Job drawing, mm, ordinate dimensions from the low corner. One solid piece. A direction names the side the tool comes from. Give positions to 0.01 mm unless a question says otherwise; leave off trailing zeros. Write each loop counter-clockwise with the first axis right and the second up, starting at its lowest first coordinate (ties: lowest second). Pieces come first, ordered by that corner, then holes. Notation, with made-up numbers: (-2, -7.5) -> (31, -7.5) arc R13 cw to (31, 17.5) -> close; hole circle Ø10 at (5, 22). An arc over 180 degrees is marked (long way). Put each result on its own line as item: value. Start each with the question number.
Item 1: Flat gauge pins, fed straight in: pin 1 Ø4 at (y, z) = (9, 18.5) entering from -X; pin 2 Ø1.9 at (x, z) = (34, 19) entering from -Y; pin 3 Ø1 at (x, z) = (14.5, 12.5) entering from -Y. Where does each tip first touch, or does it go through?
Item 2: Slice it at A-A, the plane x = 3.81. List the corners of the cut face in (y, z) (1 decimal).
Item 3: Two-plate mould, pull along X, no slides. Class the marked faces 3, 4 and 5: pulls with the +X half, pulls with the -X half, needs draft (parallel to the pull), parting line crosses it, or undercut.
Item 4: Slice it at B-B, the plane z = 15.5. List the corners of the cut face in (x, y).
Item 5: Slice it at C-C, the plane y = 5. Give the number of separate pieces and of enclosed holes in the cut face.
Item 6: Tool access for the marked faces 1 and 2: list every direction of +Z, -Z, +X, -X, +Y, -Y with a clear straight run to the whole face (end or side of a thin tool).
Item 7: Drill centre lines: line 1 along Z through (x, y) = (16, 2.75) (1 decimal); line 2 along Z through (x, y) = (3.81, 14) (1 decimal); line 3 along X through (y, z) = (6.5, 22.75). Where is each one in solid material? Low to high.
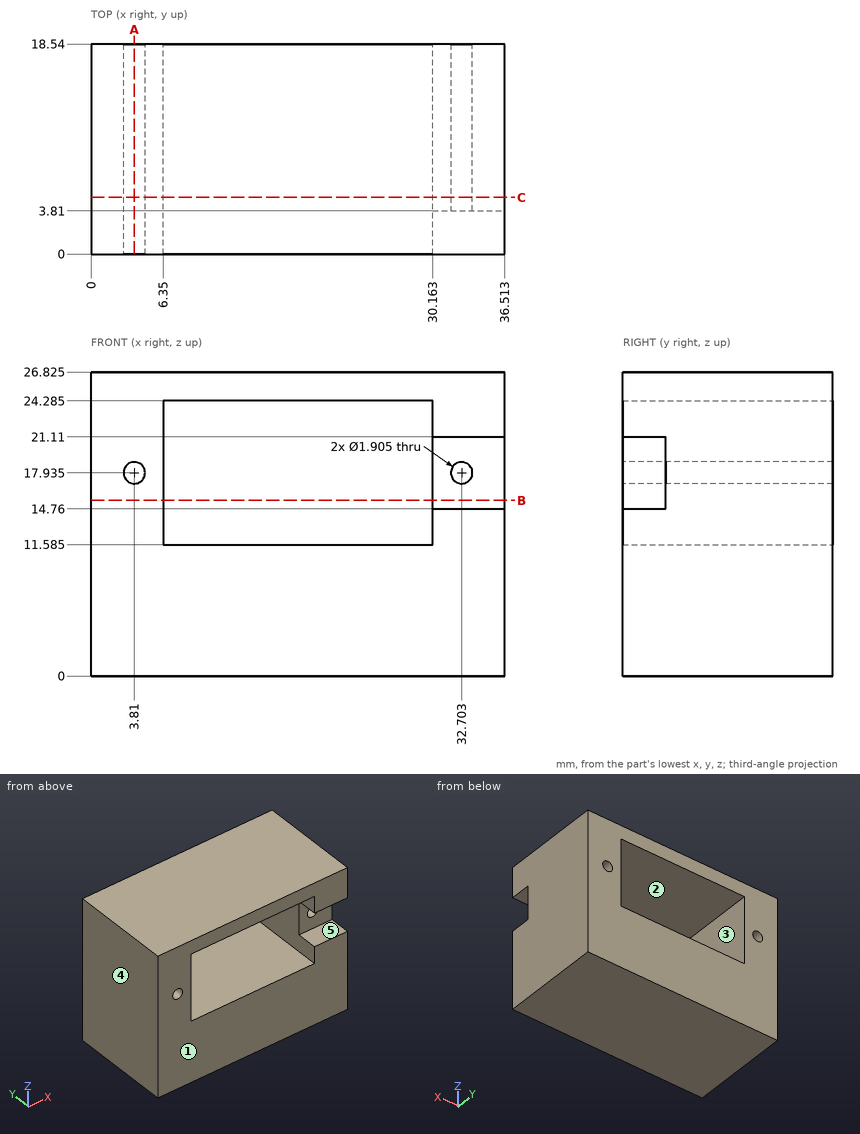
Values follow:
1. pin 1: x = 0
1. pin 2: y = 3.81
1. pin 3: through
2. outline: (0, 0) -> (18.5, 0) -> (18.5, 17) -> (0, 17) -> close; (0, 18.9) -> (18.5, 18.9) -> (18.5, 26.8) -> (0, 26.8) -> close
3. face 3: undercut
3. face 4: pulls with the -X half
3. face 5: needs draft
4. outline: (0, 0) -> (6.35, 0) -> (6.35, 18.54) -> (0, 18.54) -> close; (30.16, 3.81) -> (36.51, 3.81) -> (36.51, 18.54) -> (30.16, 18.54) -> close
5. separate pieces: 1
5. enclosed holes: 3
6. face 1: +Z, -Z, +X, -X, -Y
6. face 2: +Y, -Y
7. line 1: 0 to 11.6, 24.3 to 26.8
7. line 2: 0 to 17, 18.9 to 26.8
7. line 3: 0 to 6.35, 30.16 to 36.51
